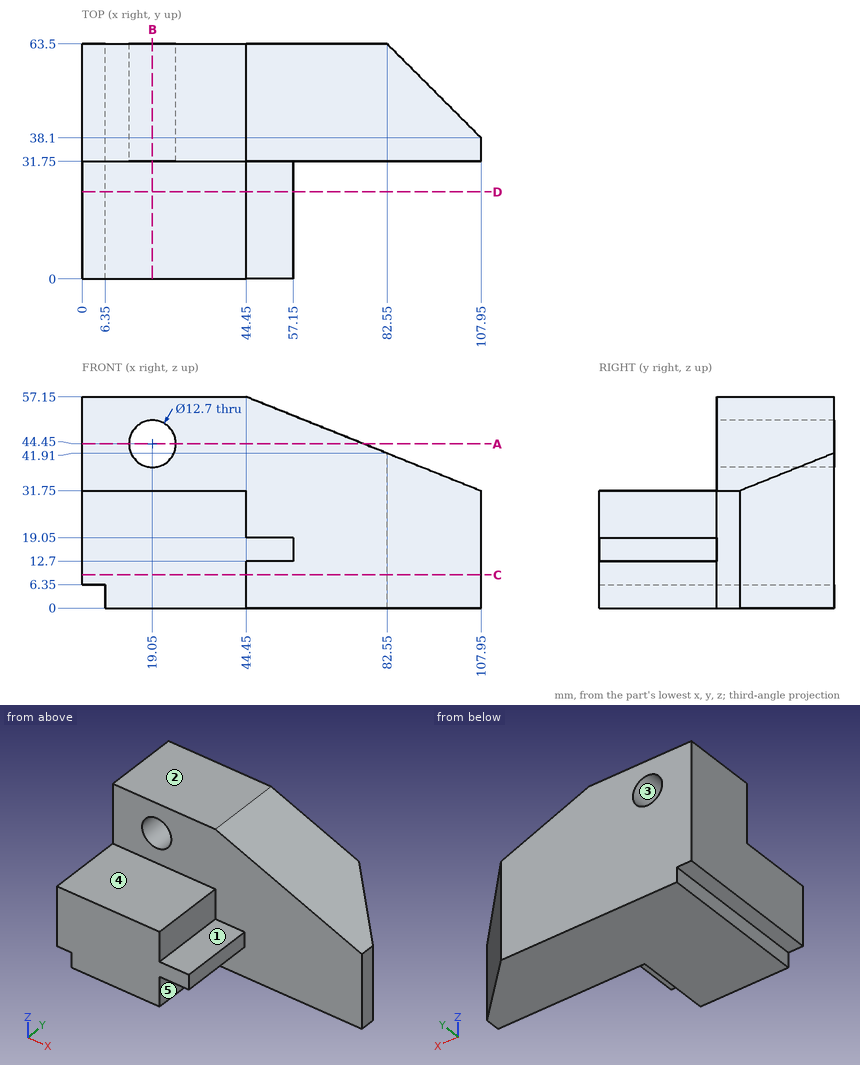
Check sheet for the drawn part. Datum: minimum x, y, z corner. Units: mm. A direction names the side the tool comes from. Round coordinates to 2 decimals unless told otherwise and drop trailing zeros. Loops run counter-clockwise (first coordinate to the right, second up) from the corner with the lowest first, then second, coordinate; pieces in that order, holes last. Notation, with made-up numbers: (2, -39.5) - (25, -39.5) arc R10 cw to (25, -35.5) - close; hole circle Ø8 at (89, 9.5). An arc over 180 degrees is marked (long way). Write item = value, one per line. Start each with the question number.
1. Section check C-C on z = 9. Enter the section's corners in (x, y), then the cut area to 3 significant figures.
2. Section check D-D on y = 23.5. Enter the section's corners in (x, z).
3. Section check A-A on z = 44.45. Enter the section's corners in (x, y), then the cut area to 3 significant figures.
4. Set-up check for the marked faces 1 and 2: record each of +Z, -Z, +X, -X, +Y, -Y from which the full face is reachable in a straight line by a thin tool's end or side.
5. Section check B-B on x = 19.05. Enter the section's corners in (y, z).
6. Depth check by flat-ended pin: pin 1 (5 mm diameter, centred on y = 23, z = 17.5, fed in from +X); pin 2 (6 mm diameter, centred on x = 71, y = 30.5, fed in from +Z); pin 3 (2 mm diameter, centred on x = 81.5, z = 18.5, fed in from -Y). Enter the tip coordinate at first touch or a pass-through.
7. Thickness scan on line 1 (Z direction, x = 19.05, y = 48); line 2 (Y direction, x = 11, z = 39); line 3 (X direction, y = 6.5, z = 2). Record the ranges inside material, lowest first.
8. Mould release check, pull along Z, two halves, no side actions. Record for the marked faces 3, 4 and 5: released by +Z, released by -Z, zero draft, split by the parting line, or undercut.
Working result:
q1.outline = (0, 0) - (44.45, 0) - (44.45, 31.75) - (107.95, 31.75) - (107.95, 38.1) - (82.55, 63.5) - (0, 63.5) - close
q1.area = 4,520 mm^2
q2.outline = (0, 6.35) - (6.35, 6.35) - (6.35, 0) - (44.45, 0) - (44.45, 12.7) - (57.15, 12.7) - (57.15, 19.05) - (44.45, 19.05) - (44.45, 31.75) - (0, 31.75) - close
q3.outline = (0, 31.75) - (12.7, 31.75) - (12.7, 63.5) - (0, 63.5) - close; (25.4, 31.75) - (76.2, 31.75) - (76.2, 63.5) - (25.4, 63.5) - close
q3.area = 2,020 mm^2
q4.face_1 = +Z, +X, -Y
q4.face_2 = +Z, +X, -X, +Y, -Y
q5.outline = (0, 0) - (63.5, 0) - (63.5, 38.1) - (31.75, 38.1) - (31.75, 31.75) - (0, 31.75) - close; (31.75, 50.8) - (63.5, 50.8) - (63.5, 57.15) - (31.75, 57.15) - close
q6.pin_1 = 57.15
q6.pin_2 = 47.62
q6.pin_3 = 31.75
q7.line_1 = 0 to 38.1, 50.8 to 57.15
q7.line_2 = 31.75 to 63.5
q7.line_3 = 6.35 to 44.45
q8.face_3 = undercut
q8.face_4 = released by +Z
q8.face_5 = zero draft
